Source: CAD feature listing. Evaluate the final solid. Frame: model axes, mm. Face numbers are marked on the shaded views. A direction names the side the tool comes from. Round coordinates to 2 decimals unless told otherwise and drop trailing zeros. Loops run counter-clockwise (first coordinate to the right, second up) from the corner with the lowest first, then second, coordinate; pieces in that order, holes last.
(1) Section A-A, the plane x = 9. Return the cut outline in (y, z).
(2) Set-up query: the marked faces 1 and 2. Return all of +Z, -Z, +X, -X, +Y, -Y with unobstructed straight access to the full face (end or side cutting, diameter ignored); none if empty.
(3) Mould query, pull axis X, two halves, no side actions, for the marked faces 3, 4 and 5. Classes: pulls with the +X half, pulls with the -X half, needs draft (parallel to the pull), parting line crosses it, or undercut.
(4) Material intervals for probe 1 along X at (y, z) = (24, 4); probe 2 along X at (y, z) = (3.5, -1.1); probe 3 along X at (y, z) = (3.5, 0.1), sorted ascending.
(5) Section B-B, the plane x = 30. Return the cut outline in (y, z).
(6) First-contact query: pin 1 Ø0.5 at (x, z) = (8, 0.5) entering from -Y; pin 2 Ø8.5 at (x, y) = (12, 18) entering from +Z; pin 3 Ø4 at (x, z) = (18.5, 20.5) entering from +Y. Flat tips, straight axial feed; report the tip coordinate or a pass-through.
(7) Section D-D, the plane x = 35.5. Return the cut outline in (y, z), plus the area to 3 significant figures.
(8) Section C-C, the plane y = 18.5. Return the cut outline in (x, z), plus the area to 3 significant figures.
```python
from build123d import *

# Parameters (mm, degrees)
F1_DEPTH = 40
F2_T     = -1
F0_W     = 30
F0_H     = 2
F3_DEPTH = 40
F4_W     = 8
F4_H     = 6
F5_DEPTH = 10
F6_R     = 1.4
F7_DEPTH = 3
F8_R     = 4


with BuildPart() as f1:
    # F0 (on Right) → F1 (new body)
    with BuildSketch(Plane.YZ):
        Polygon((10.2606042998, 28.1907786236), (0, 0), (30, 0), (12.1399895413, 27.5067383369), align=None)
    extrude(amount=F1_DEPTH)

    # F2
    f2_openings = [f1.faces().sort_by_distance(p)[0] for p in [
        (20, 21.069995, 13.753369),
    ]]
    offset(amount=F2_T, openings=f2_openings, kind=Kind.INTERSECTION)

    # F0 (on Right) → F3 (join)
    with BuildSketch(Plane.YZ):
        with Locations((15, -1)):
            Rectangle(F0_W, F0_H)
    extrude(amount=F3_DEPTH)

    # F4 (on Front) → F5 (cut)
    with BuildSketch(Plane.XZ):
        with Locations((9, 3)):
            Rectangle(F4_W, F4_H)
    extrude(amount=-F5_DEPTH, mode=Mode.SUBTRACT)

    # F6 (on face) → F7 (cut)
    with BuildSketch(Plane(origin=(0, 0, -2), x_dir=(1, 0, 0), z_dir=(0, 0, -1))):
        with Locations((4.75, -3.5)):
            Circle(F6_R)
        with Locations((35.25, -3.5)):
            Circle(F6_R)
    extrude(amount=-F7_DEPTH, mode=Mode.SUBTRACT)

    # F8
    f8_edges = [f1.edges().sort_by_distance(p)[0] for p in [
        (1, 6.143212, 13.954533),
        (39, 6.143212, 13.954533),
        (0, 5.130302, 14.095389),
        (40, 5.130302, 14.095389),
    ]]
    fillet(f8_edges, radius=F8_R)


solid = f1.part
```
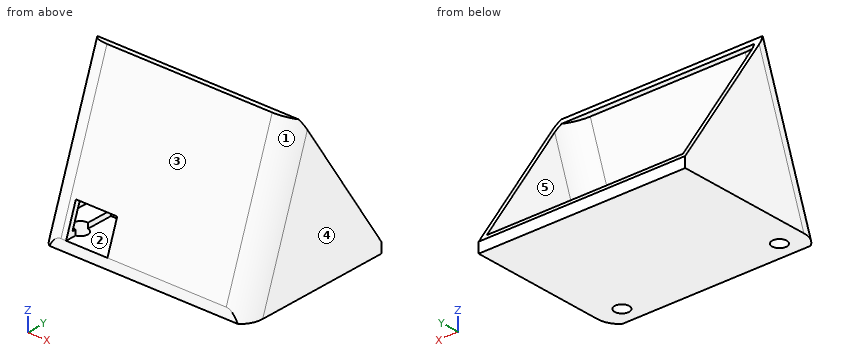
Output values:
1. outline: (0, -2) - (30, -2) - (30, 0) - (29.35, 1) - (10, 1) - (10, 0) - (0, 0) - close; (2.18, 6) - (3.25, 6) - (10.86, 26.91) - (13.04, 26.11) - (12.14, 27.51) - (10.26, 28.19) - close
2. face 1: +Z, +X, -Y
2. face 2: -Y
3. face 3: needs draft
3. face 4: pulls with the +X half
3. face 5: undercut
4. probe 1: x = 0 to 1, 39 to 40
4. probe 2: x = 0.01 to 3.35, 6.15 to 33.85, 36.65 to 39.99
4. probe 3: x = 0.07 to 3.35, 13 to 33.85, 36.65 to 39.93
5. outline: (0, -2) - (30, -2) - (30, 0) - (29.35, 1) - (1.43, 1) - (10.86, 26.91) - (13.04, 26.11) - (12.14, 27.51) - (10.26, 28.19) - (0, 0) - close
6. pin 1: stops at y = 10
6. pin 2: stops at z = 1
6. pin 3: stops at y = 9.25
7. outline: (0, -2) - (2.12, -2) - (2.12, 1) - (1.46, 1) - (10.89, 26.9) - (13.04, 26.11) - (12.14, 27.51) - (10.26, 28.19) - (0, 0) - close; (4.88, -2) - (30, -2) - (30, 0) - (29.35, 1) - (4.88, 1) - close
7. area: 113 mm2
8. outline: (0, -2) - (40, -2) - (40, 17.71) - (39, 17.71) - (39, 1) - (1, 1) - (1, 17.71) - (0, 17.71) - close
8. area: 153 mm2
